The drawing under review shows one solid part. Ordinate dimensions are in mm from its lowest x, y, z. Give positions to 0.01 mm unless a question says otherwise; leave off trailing zeros. Order: outer loops, then holes, each group sorted by start corner. A loop starts at its lowest first (then second) coordinate and runs counter-clockwise, first axis right, second up. Notation, with made-up numbers: (36.25, 41) - (48.25, 41) arc R27 cw to (48.25, 74) - close; hole circle Ø6 at (18.25, 49). An arc over 180 degrees is marked (long way). Use CSV: the item, a comma, the result in double quotes.
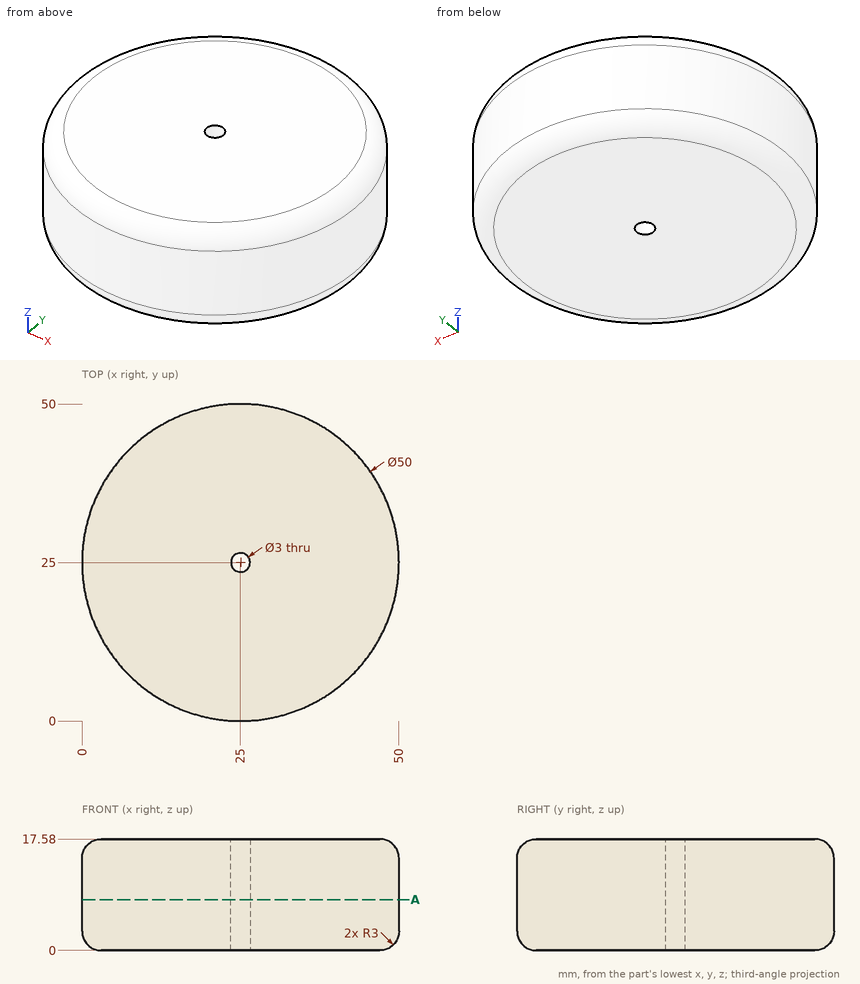
Item 1: Wall thickness on L1, parallel to Y at x = 25, z = 7.25; L2, parallel to X at y = 44.5, z = 15.25; L3, parallel to X at y = 19.5, z = 12.5: over which ranges is each line inside the solid? List them lowest first.
Results list:
L1,"y = 0 to 23.5, 26.5 to 50"
L2,"x = 9.48 to 40.52"
L3,"x = 0.61 to 49.39"
Item 2: Take a section at A-A, the plane z = 8. Give the boundary of the cut face in (x, y).
Results list:
outline,"circle Ø50 at (25, 25); hole circle Ø3 at (25, 25)"
Item 3: Clearance check with flat-ended pins moving along their axes: pin 1 (8 mm diameter, centred on x = 9.5, z = 6.5, fed in from +Y); pin 2 (8 mm diameter, centred on x = 8.5, z = 4, fed in from +Y); pin 3 (1.5 mm diameter, centred on x = 22.5, z = 6.5, fed in from +Y). State where each tip first meets the part, or that it passes through.
Results list:
pin 1,"stops at y = 47.2"
pin 2,"stops at y = 46.65"
pin 3,"stops at y = 49.94"
